```python
from build123d import *

# Parameters (mm, degrees)
SKETCH1_W           = 68.58
SKETCH1_H           = 43.434
BOSS_EXTRUDE1_DEPTH = 5.08
SKETCH2_W           = 43.434
SKETCH2_H           = 5.08
BOSS_EXTRUDE2_DEPTH = 25.4
SKETCH3_W           = 25.4
SKETCH3_H           = 6.35
BOSS_EXTRUDE3_DEPTH = 37.592


with BuildPart() as part:
    # Sketch1 → Boss-Extrude1 (new body)
    with BuildSketch(Plane(origin=(0, 0, 0), x_dir=(0, 1, 0), z_dir=(0, 0, 1))):
        with Locations((34.29, 21.717)):
            Rectangle(SKETCH1_W, SKETCH1_H)
    extrude(amount=BOSS_EXTRUDE1_DEPTH)

    # Sketch2 → Boss-Extrude2 (add)
    with BuildSketch(Plane.XY.offset(5.08)):
        with Locations((-21.717, 8.128)):
            Rectangle(SKETCH2_W, SKETCH2_H)
        with Locations((-21.717, 60.452)):
            Rectangle(SKETCH2_W, SKETCH2_H)
    extrude(amount=BOSS_EXTRUDE2_DEPTH)

    # Sketch3 → Boss-Extrude3 (add)
    with BuildSketch(Plane.XY.offset(5.08)):
        with Locations((-13.716, 34.29)):
            Rectangle(SKETCH3_W, SKETCH3_H)
    extrude(amount=BOSS_EXTRUDE3_DEPTH)


solid = part.part
```
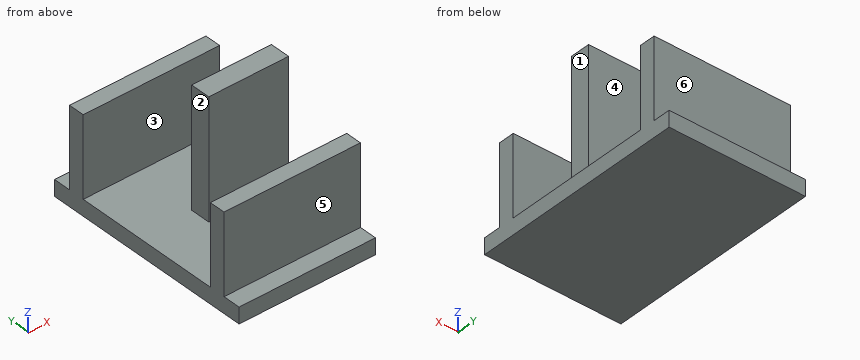
Could you check a few things on this model? Use its own coordinates, in mm. Face numbers are marked on the shaded views. A direction names the side the tool comes from. Give positions to 0.01 mm unless a question says otherwise; leave off trailing zeros. Write each loop counter-clockwise with the first axis right and the second up, starting at its lowest first coordinate (ties: lowest second). Pieces come first, ordered by that corner, then holes. Notation, with made-up numbers: (-29, 89) - (22, 89) arc R13 cw to (22, 97) - close; hole circle Ø7 at (-11.5, 7). An arc over 180 degrees is marked (long way). One line per item, written item: value. Start each with the question number.
Item 1: Imagine slicing it at A-A, the plane z = 18.5. List the corners of the cut face in (x, y) for me (3 decimals), and give its area (3 significant figures).
Item 2: Please list where these lines run through material, in increasing order: line 1 (Y direction, x = -16, z = 10) (3 decimals); line 2 (Y direction, x = -37.5, z = 24.5); line 3 (Z direction, x = -28, y = 31). Write a range as from..to.
Item 3: Imagine slicing it at B-B, the plane x = -15. List the corners of the cut face in (y, z) for me (3 decimals), and give its area (3 significant figures).
Item 4: Imagine slicing it at D-D, the plane x = -30. List the corners of the cut face in (y, z) for me.
Item 5: Imagine slicing it at C-C, the plane y = 61. List the corners of the cut face in (x, z) for me.
Item 6: Which directions (+Z, -Z, +X, -X, +Y, -Y) give clear straight access to the entire face, cutting with the end or side of a thin tool? Please do the marked faces 1, 2 and 3.
Item 7: I'm going to push flat-ended pins straight in: pin 1 (12.5 mm diameter, centred on x = -29, z = 18, fed in from +Y); pin 2 (4 mm diameter, centred on x = -20, y = 7.5, fed in from +Z); pin 3 (13 mm diameter, centred on x = -31.5, y = 37.5, fed in from +Z); pin 4 (3 mm diameter, centred on y = 34.5, z = 31.5, fed in from -X). Where does each tip first touch, or does it pass through?
Item 8: If we mould it in two halves opening along Y, with no side actions, what happens to the marked faces 4, 5 and 6? For each: +Y half, -Y half, draft (parallel to the pull), parting line (faces both ways), or undercut.
Geometry says:
1. outline: (-43.434, 5.588) - (0, 5.588) - (0, 10.668) - (-43.434, 10.668) - close; (-43.434, 57.912) - (0, 57.912) - (0, 62.992) - (-43.434, 62.992) - close; (-26.416, 31.115) - (-1.016, 31.115) - (-1.016, 37.465) - (-26.416, 37.465) - close
1. area: 603 mm^2
2. line 1: 5.588..10.668, 31.115..37.465, 57.912..62.992
2. line 2: 5.59..10.67, 57.91..62.99
2. line 3: 0..5.08
3. outline: (0, 0) - (68.58, 0) - (68.58, 5.08) - (62.992, 5.08) - (62.992, 30.48) - (57.912, 30.48) - (57.912, 5.08) - (37.465, 5.08) - (37.465, 42.672) - (31.115, 42.672) - (31.115, 5.08) - (10.668, 5.08) - (10.668, 30.48) - (5.588, 30.48) - (5.588, 5.08) - (0, 5.08) - close
3. area: 845 mm^2
4. outline: (0, 0) - (68.58, 0) - (68.58, 5.08) - (62.99, 5.08) - (62.99, 30.48) - (57.91, 30.48) - (57.91, 5.08) - (10.67, 5.08) - (10.67, 30.48) - (5.59, 30.48) - (5.59, 5.08) - (0, 5.08) - close
5. outline: (-43.43, 0) - (0, 0) - (0, 30.48) - (-43.43, 30.48) - close
6. face 1: +Z, +X
6. face 2: +Z, -X
6. face 3: +Z, +X, -X
7. pin 1: y = 62.99
7. pin 2: z = 30.48
7. pin 3: z = 42.67
7. pin 4: x = -26.42
8. face 4: undercut
8. face 5: -Y half
8. face 6: +Y half
